Work out the finished part from the listing and answer in its coordinate system (mm). Face numbers are marked on the shaded views. Round coordinates to 2 decimals unless told otherwise and drop trailing zeros. Order: outer loops, then holes, each group sorted by start corner. A loop starts at its lowest first (then second) coordinate and runs counter-clockwise, first axis right, second up. Notation, with made-up numbers: (-0.5, 0.5) - (48.5, 0.5) arc R14 cw to (48.5, 19.5) - close; hole circle Ø1 at (37.25, 88.5). An arc over 180 degrees is marked (long way). Use one line per item in the form item = value. Start each with the question number.
Q1. Given P1, Ø18, axis at x = -75, y = 25, coming from the -Z side; P2, Ø3, axis at y = 41, z = 11, coming from the +X side; P3, Ø3, axis at x = 8.5, z = 10, coming from the -Y side; P4, Ø8, axis at y = 3, z = 12, coming from the -X side, each flat-ended and moving along its own axis, determine where each tip first touches the part or whether it passes through.
Q2. The part is cut by section C-C on y = 108. Determine the outline of the cut face in (x, z), plus the area to 4 significant figures.
Q3. Find the intervals of material crossed by line 1 (Y direction, x = -75, z = 2.65); line 2 (Y direction, x = -25.5, z = 9.75); line 3 (X direction, y = 6, z = 13.5), in increasing order. Write a range as [from, to].
Q4. The part is cut by section B-B on y = -125. Determine the outline of the cut face in (x, z), plus the area to 3 significant figures.
Q5. The part is cut by section A-A on x = -125. Determine the outline of the cut face in (y, z).
Q6. The part is cut by section D-D on z = 7.25. State how many separate pieces and enclosed holes the cut face has, plus the area to 3 significant figures.
Q7. For a pull along Y with two mould halves and no side action, classify the marked faces 1 and 2 as +Y half, -Y half, draft (parallel to the pull), parting line (faces both ways), or undercut.
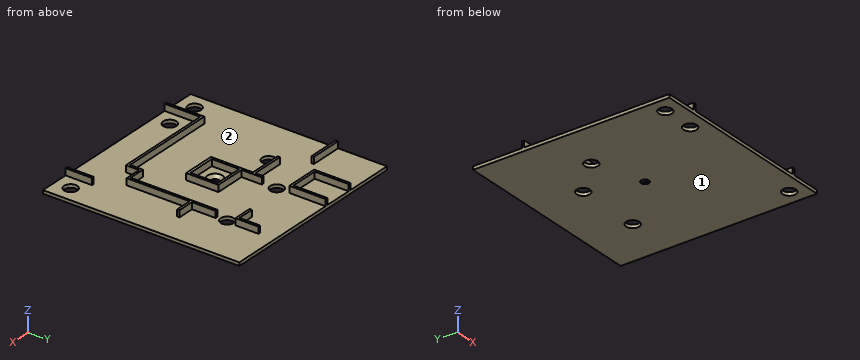
from build123d import *

# Parameters (mm, degrees)
SKETCH3_W           = 298
SKETCH3_H           = 298
BOSS_EXTRUDE2_DEPTH = 5
SKETCH4_R           = 10
CUT_EXTRUDE5_DEPTH  = 56
SKETCH5_W           = 43
SKETCH5_H           = 3.5
SKETCH5_W_2         = 49
SKETCH5_W_3         = 3.5
SKETCH5_H_2         = 49.019827061
SKETCH5_H_3         = 4.008691654
SKETCH5_W_4         = 25
SKETCH5_H_4         = 35
SKETCH5_H_5         = 16.5
SKETCH5_H_6         = 40
SKETCH5_W_5         = 50
BOSS_EXTRUDE6_DEPTH = 10


with BuildPart() as part:
    # Sketch3 → Boss-Extrude2 (new body)
    with BuildSketch(Plane.XY):
        Rectangle(SKETCH3_W, SKETCH3_H)
    extrude(amount=BOSS_EXTRUDE2_DEPTH)

    # Sketch4 → Cut-Extrude5 (cut)
    with BuildSketch(Plane.XY.offset(5)):
        with Locations((-75, 25)):
            Circle(SKETCH4_R)
        with Locations((-25, 75)):
            Circle(SKETCH4_R)
        with Locations((75, 75)):
            Circle(SKETCH4_R)
        with Locations((-75, -125)):
            Circle(SKETCH4_R)
        with Locations((-125, -125)):
            Circle(SKETCH4_R)
        with Locations((125, -125)):
            Circle(SKETCH4_R)
    extrude(amount=-CUT_EXTRUDE5_DEPTH, mode=Mode.SUBTRACT)

    # Sketch5 → Boss-Extrude6 (add)
    with BuildSketch(Plane.XY.offset(5)):
        Polygon((-71.5, 149), (-75, 149), (-75, 94), (-71.5, 94), (-71.5, 97.5), align=None)
        with Locations((-50, 95.75)):
            Rectangle(SKETCH5_W, SKETCH5_H)
        Polygon((-25, 149), (-28.5, 149), (-28.5, 97.5), (-28.5, 94), (-25, 94), align=None)
        with Locations((-124.5, 73.095100697)):
            Rectangle(SKETCH5_W_2, SKETCH5_H)
        Polygon((-25, 38.670579352), (-25, 24.019827061), (-21.5, 24.019827061), (-21.5, 55.019827061), (-25, 55.019827061), (-25, 42.170579352), align=None)
        with Locations((-23.25, -0.490086469)):
            Rectangle(SKETCH5_W_3, SKETCH5_H_2)
        with Locations((0, 22.269827061)):
            Rectangle(SKETCH5_W, SKETCH5_H)
        with Locations((23.25, -0.490086469)):
            Rectangle(SKETCH5_W_3, SKETCH5_H_2)
        with Locations((0, -22.995654173)):
            Rectangle(SKETCH5_W, SKETCH5_H_3)
        Polygon((75, -71.842185644), (75, -75), (78.5, -75), (78.5, 20.519827061), (78.5, 24.019827061), (78.5, 60), (75, 60), align=None)
        with Locations((91, 22.269827061)):
            Rectangle(SKETCH5_W_4, SKETCH5_H)
        with Locations((76.75, 107.5)):
            Rectangle(SKETCH5_W_3, SKETCH5_H_4)
        with Locations((62.5, 91.75)):
            Rectangle(SKETCH5_W_4, SKETCH5_H)
        Polygon((50, -71.842185644), (50, -75), (53.5, -75), (75, -75), (75, -71.842185644), align=None)
        with Locations((51.75, -83.25)):
            Rectangle(SKETCH5_W_3, SKETCH5_H_5)
        Polygon((-96.5, -91.5), (-96.5, -95), (53.5, -95), (53.5, -91.5), (50, -91.5), align=None)
        Polygon((-100, -91.5), (-100, -149), (-96.5, -149), (-96.5, -95), (-96.5, -91.5), align=None)
        with Locations((101.75, -129)):
            Rectangle(SKETCH5_W_3, SKETCH5_H_6)
        with Locations((-50, 40.420579352)):
            Rectangle(SKETCH5_W_5, SKETCH5_H)
    extrude(amount=BOSS_EXTRUDE6_DEPTH)

    # Sketch7 → CSK for 7/16 Flat Head Machine Screw (100)1 (revolve, cut)
    with BuildSketch(Plane(origin=(0, 0, 5), x_dir=(0, -1, 0), z_dir=(1, 0, 0))):
        Polygon((0, 0), (0, 5), (5.95249, 5), (5.95249, 4.489610968), (11.303, 0), align=None)
    revolve(axis=Axis((0, 0, 11.35), (0, 0, -1)), mode=Mode.SUBTRACT)


solid = part.part
Found:
q1.P1 = through
q1.P2 = 78.5
q1.P3 = -95
q1.P4 = -25
q2.outline = (-149, 0) - (149, 0) - (149, 5) - (78.5, 5) - (78.5, 15) - (75, 15) - (75, 5) - (-25, 5) - (-25, 15) - (-28.5, 15) - (-28.5, 5) - (-71.5, 5) - (-71.5, 15) - (-75, 15) - (-75, 5) - (-149, 5) - close
q2.area = 1,595 mm²
q3.line_1 = [-149, -135], [-115, 15], [35, 149]
q3.line_2 = [-95, -91.5], [38.67, 42.17], [94, 149]
q3.line_3 = [-25, -21.5], [21.5, 25], [75, 78.5]
q4.outline = (-149, 0) - (-135, 0) - (-135, 5) - (-149, 5) - close; (-115, 0) - (-85, 0) - (-85, 5) - (-96.5, 5) - (-96.5, 15) - (-100, 15) - (-100, 5) - (-115, 5) - close; (-65, 0) - (115, 0) - (115, 5) - (103.5, 5) - (103.5, 15) - (100, 15) - (100, 5) - (-65, 5) - close; (135, 0) - (149, 0) - (149, 5) - (135, 5) - close
q4.area = 1,260 mm²
q5.outline = (-149, 0) - (-135, 0) - (-135, 5) - (-149, 5) - close; (-115, 0) - (149, 0) - (149, 5) - (74.85, 5) - (74.85, 15) - (71.35, 15) - (71.35, 5) - (-115, 5) - close
q6.separate_pieces = 6
q6.enclosed_holes = 1
q6.area = 3,430 mm²
q7.face_1 = draft
q7.face_2 = undercut
